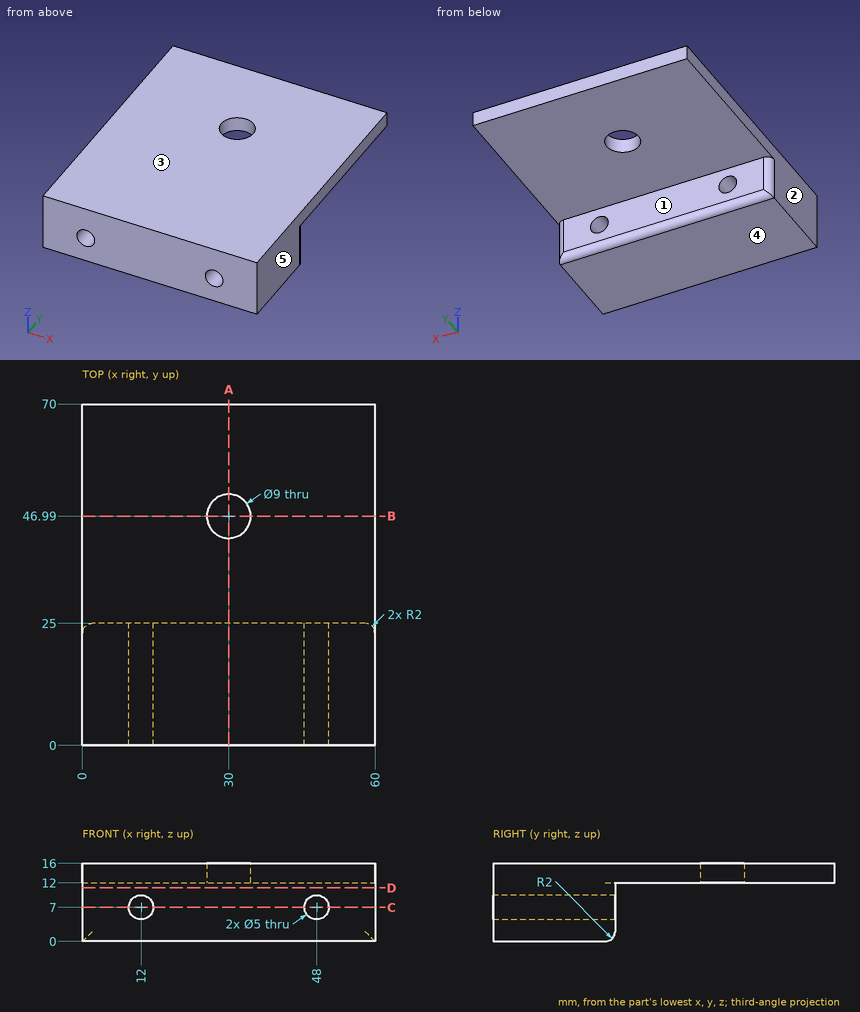
Input: dimensioned drawing with shaded views. Units: mm. Origin: part minimum x, y, z. A direction names the side the tool comes from. Coordinates: 2 decimals unless noted, no trailing zeros. Order: outer loops, then holes, each group sorted by start corner. A loop starts at its lowest first (then second) coordinate and runs counter-clockwise, first axis right, second up. Notation, with made-up numbers: (48.25, 28) - (101.25, 28) arc R11 ccw to (101.25, 36) - close; hole circle Ø10 at (-13.75, 67). An arc over 180 degrees is marked (long way). Return JSON: item names as keys, results as strings. Group by question number.
1. Cut plane C-C (z = 7). Output: boundary loops of the cut face in (x, y), plus the area to 3 significant figures.
2. Material intervals for line 1 along X through (y, z) = (15.5, 6.25); line 2 along Y through (x, z) = (30, 13.9); line 3 along Z through (x, y) = (30.5, 33), sorted ascending. Write a range as [from, to].
3. Pin query (flat end, axial travel): pin 1 (8 mm diameter, centred on x = 16, y = 44, fed in from -Z); pin 2 (5 mm diameter, centred on x = 16.5, z = 6, fed in from +Y); pin 3 (5.5 mm diameter, centred on x = 30, y = 46.99, fed in from +Z). Return the tip coordinate at first contact, or that it passes through.
4. Cut plane B-B (y = 46.99). Output: boundary loops of the cut face in (x, z), plus the area to 3 significant figures.
5. Cut plane D-D (z = 11). Output: boundary loops of the cut face in (x, y), plus the area to 3 significant figures.
6. Pull-direction query (Z, two-part tool) for the marked faces 3, 4 and 5; classes: pulls with the +Z half, pulls with the -Z half, needs draft (parallel to the pull), parting line crosses it, or undercut.
7. Set-up query: the marked faces 1 and 2. Return all of +Z, -Z, +X, -X, +Y, -Y with unobstructed straight access to the full face (end or side cutting, diameter ignored); none if empty.
8. Cut plane A-A (x = 30). Output: boundary loops of the cut face in (y, z), plus the area to 3 significant figures.
Resolved:
{
 "1": {"outline": "(0, 0) - (9.5, 0) - (9.5, 25) - (2, 25) arc R2 ccw to (0, 23) - close; (14.5, 0) - (45.5, 0) - (45.5, 25) - (14.5, 25) - close; (50.5, 0) - (60, 0) - (60, 23) arc R2 ccw to (58, 25) - (50.5, 25) - close", "area": "1,250 mm²"},
 "2": {"line 1": "x = [0, 9.62], [14.38, 45.62], [50.38, 60]", "line 2": "y = [0, 42.49], [51.49, 70]", "line 3": "z = [12, 16]"},
 "3": {"pin 1": "stops at z = 12", "pin 2": "stops at y = 25", "pin 3": "passes through"},
 "4": {"outline": "(0, 12) - (25.5, 12) - (25.5, 16) - (0, 16) - close; (34.5, 12) - (60, 12) - (60, 16) - (34.5, 16) - close", "area": "204 mm²"},
 "5": {"outline": "(0, 0) - (60, 0) - (60, 23) arc R2 ccw to (58, 25) - (2, 25) arc R2 ccw to (0, 23) - close", "area": "1,500 mm²"},
 "6": {"face 3": "pulls with the +Z half", "face 4": "pulls with the -Z half", "face 5": "needs draft"},
 "7": {"face 1": "-Z, +X, -X, +Y", "face 2": "+Z, -Z, -X, +Y, -Y"},
 "8": {"outline": "(0, 0) - (23, 0) arc R2 ccw to (25, 2) - (25, 12) - (42.49, 12) - (42.49, 16) - (0, 16) - close; (51.49, 12) - (70, 12) - (70, 16) - (51.49, 16) - close", "area": "543 mm²"}
}
